Design review of the part built by this model. Coordinates are the model's own, in mm. A direction names the side the tool comes from. Coordinates: 2 decimals unless noted, no trailing zeros.
Q1. Insertion check: pin 1 (12 mm diameter, centred on x = -9, z = 16.5, fed in from -Y); pin 2 (1.5 mm diameter, centred on y = 9, z = 27.5, fed in from +X); pin 3 (6 mm diameter, centred on x = 2, z = 22, fed in from -Y); pin 4 (2 mm diameter, centred on x = 1.5, y = 4, fed in from -Z). Each pin has a flat end and moves straight along its axis. Give the tip position at first contact, or say it passes through.
Q2. Mouldability with a two-part tool opening along X and no side actions: class faces 4 (the flat face through (15, 5, 57.15)), 5 (the flat face through (-11.214, -11.287, 54.019)), 6 (the cylindrical face through (7.481, 10.263, 54.019)) as pulls with the +X half, pulls with the -X half, needs draft (parallel to the pull), parting line crosses it, or undercut.
Q3. For probe 1 along Z at (x, y) = (-6, -1); probe 2 along X at (y, z) = (3.5, 50.5); probe 3 along Z at (x, y) = (-7.5, -16), list the stretches that pass through material, from the lowest coordinate up.
Q4. Machinability: for faces 1 (the flat face through (-16, -2.54, 54)), 2 (the cylindrical face through (7.449, -10.286, 54.019)), 3 (the flat face through (-7.241, -14.067, 54.019)), which of the approach directions +Z, -Z, +X, -X, +Y, -Y give a long, thin tool a straight path to every point of the face, cutting with its end or side? Answer none if there is none.
```python
from build123d import *

# Parameters (mm, degrees)
F0_W     = 19.05
F0_H     = 10.16
F2_R     = 12.7
F3_DEPTH = 6.35
F4_W     = 7.2063849882
F4_H     = 5.08
F5_DEPTH = 6.35


with BuildPart() as f1:
    # F0 (on Front) → F1 (revolve)
    with BuildSketch(Plane.XZ):
        with BuildLine():
            Line((0, 46.99), (0, 0))
            Line((0, 0), (19.05, 0))
            Line((19.05, 0), (19.05, 6.985))
            add(Edge.make_bspline(
                [(19.05, 6.985), (16.2391823394, 8.5810058703), (12.6188776664, 16.288597078), (10.9922878006, 22.0505625493), (10.305692607, 30.1006807739), (11.6872230365, 34.2073674129), (13.795029925, 38.6193750914), (15.9890974554, 42.3022760514), (18.1140442061, 45.4568990599), (19.05, 46.99)],
                knots=[0, 0, 0, 0, 0.1903034554, 0.3390772007, 0.4978932907, 0.618503958, 0.7432602735, 0.8640913793, 1, 1, 1, 1], degree=3))
            Line((19.05, 46.99), (0, 46.99))
        make_face()
        with Locations((9.525, 52.07)):
            Rectangle(F0_W, F0_H)
    revolve(axis=Axis((0, 0, 28.575), (0, 0, 1)))

    # F2 (on face) → F3 (cut)
    with BuildSketch(Plane.XY.offset(57.15)):
        Circle(F2_R)
    extrude(amount=-F3_DEPTH, mode=Mode.SUBTRACT)

    # F4 (on face) → F5 (cut)
    with BuildSketch(Plane.XY.offset(57.15)):
        with Locations((16.0466003874, 0)):
            Rectangle(F4_W, F4_H)
        Polygon((14.4040418363, 13.6047616321), (8.5739539128, 9.3689548137), (11.5599029945, 5.2591484823), (17.3899909179, 9.4949553006), align=None)
        Polygon((3.6564363849, 19.4729667295), (1.4295409556, 12.6192873276), (6.2609080584, 11.0494809962), (8.4878034877, 17.9031603981), align=None)
        Polygon((-8.4878034877, 17.9031603981), (-6.2609080584, 11.0494809962), (-1.4295409556, 12.6192873276), (-3.6564363849, 19.4729667295), align=None)
        Polygon((-17.3899909179, 9.4949553006), (-11.5599029945, 5.2591484823), (-8.5739539128, 9.3689548137), (-14.4040418363, 13.6047616321), align=None)
        with Locations((-16.0466003874, 0)):
            Rectangle(F4_W, F4_H)
        Polygon((-14.4040418363, -13.6047616321), (-8.5739539128, -9.3689548137), (-11.5599029945, -5.2591484823), (-17.3899909179, -9.4949553006), align=None)
        Polygon((-3.6564363849, -19.4729667295), (-1.4295409556, -12.6192873276), (-6.2609080584, -11.0494809962), (-8.4878034877, -17.9031603981), align=None)
        Polygon((8.4878034877, -17.9031603981), (6.2609080584, -11.0494809962), (1.4295409556, -12.6192873276), (3.6564363849, -19.4729667295), align=None)
        Polygon((17.3899909179, -9.4949553006), (11.5599029945, -5.2591484823), (8.5739539128, -9.3689548137), (14.4040418363, -13.6047616321), align=None)
    extrude(amount=-F5_DEPTH, mode=Mode.SUBTRACT)


solid = f1.part
```
Response:
1. pin 1: stops at y = -13.98
1. pin 2: stops at x = 6.72
1. pin 3: stops at y = -11.83
1. pin 4: stops at z = 0
2. face 4: needs draft
2. face 5: pulls with the -X half
2. face 6: undercut
3. probe 1: z = 0 to 50.8
3. probe 2: x = -18.73 to 18.73
3. probe 3: z = 0 to 8.03, 44.81 to 50.8
4. face 1: +Z, +X, -X
4. face 2: +Z
4. face 3: +Z, -Y
